Design review of the part built by this model. Coordinates are the model's own, in mm. Coordinates: 2 decimals unless noted, no trailing zeros. Loops run counter-clockwise (first coordinate to the right, second up) from the corner with the lowest first, then second, coordinate; pieces in that order, holes last. Notation, with made-up numbers: (-34.75, 45.5) - (-11.75, 45.5) arc R17 cw to (-11.75, 60.5) - close; hole circle Ø5 at (-27.5, 89.25). An arc over 180 degrees is marked (long way). Answer in a Markdown table with one row per item. Add a question column.
(1) We need section A-A, the plane z = 1.25. Write out the cut boundary in (x, y), plus the area to 3 significant figures.
(2) To check wall thickness, follow L1, parallel to Y at x = 85.5, z = 1.1; L2, parallel to Y at x = -42.5, z = 1.05; L3, parallel to Y at x = 0, z = 0.75. State the ranges of each line that lie inside material, in increasing order. Write a range as [from, to].
(3) We need section B-B, the plane y = -7.5. Write out the cut boundary in (x, z).
(4) We need section D-D, the plane x = 84. Write out the cut boundary in (y, z).
(5) We need section C-C, the plane x = -42.5. Write out the cut boundary in (y, z).
from build123d import *

# Parameters (mm, degrees)
F0_R     = 2.5
F1_DEPTH = 2


with BuildPart() as f1:
    # F0 (on Top) → F1 (new body)
    with BuildSketch(Plane.XY):
        with BuildLine():
            ThreePointArc((-2.116247, -14.695241), (-1.069039, -14.923419), (0, -15))
            Line((0, -15), (100, -15))
            ThreePointArc((100, -15), (107.5, -7.5), (100, 0))
            Line((100, 0), (1.24576, -0.048733))
            Line((1.24576, -0.048733), (-40.383753, 12.195241))
            ThreePointArc((-40.383753, 12.195241), (-49.695241, 7.116247), (-44.616247, -2.195241))
            Line((-44.616247, -2.195241), (-2.116247, -14.695241))
        make_face()
        with Locations((0, -7.5)):
            Circle(F0_R, mode=Mode.SUBTRACT)
        with Locations((-42.5, 5)):
            Circle(F0_R, mode=Mode.SUBTRACT)
    extrude(amount=F1_DEPTH)


solid = f1.part
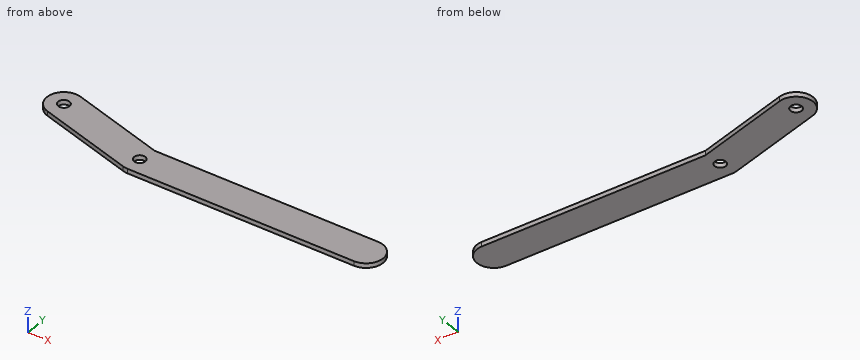
Responses:
| question | item | result |
|---|---|---|
| 1 | outline | (-44.62, -2.2) - (-2.12, -14.7) arc R7.5 ccw to (0, -15) - (100, -15) arc R7.5 ccw to (100, 0) - (1.25, -0.05) - (-40.38, 12.2) arc R7.5 ccw to start; hole circle Ø5 at (-42.5, 5); hole circle Ø5 at (0, -7.5) |
| 1 | area | 2,300 mm2 |
| 2 | L1 | y = [-15, -0.01] |
| 2 | L2 | y = [-2.82, 2.5], [7.5, 12.5] |
| 2 | L3 | y = [-15, -10], [-5, 0.32] |
| 3 | outline | (-26.58, 0) - (-2.5, 0) - (-2.5, 2) - (-26.58, 2) - close; (2.5, 0) - (107.5, 0) - (107.5, 2) - (2.5, 2) - close |
| 4 | outline | (-15, 0) - (-0.01, 0) - (-0.01, 2) - (-15, 2) - close |
| 5 | outline | (-2.82, 0) - (2.5, 0) - (2.5, 2) - (-2.82, 2) - close; (7.5, 0) - (12.5, 0) - (12.5, 2) - (7.5, 2) - close |
